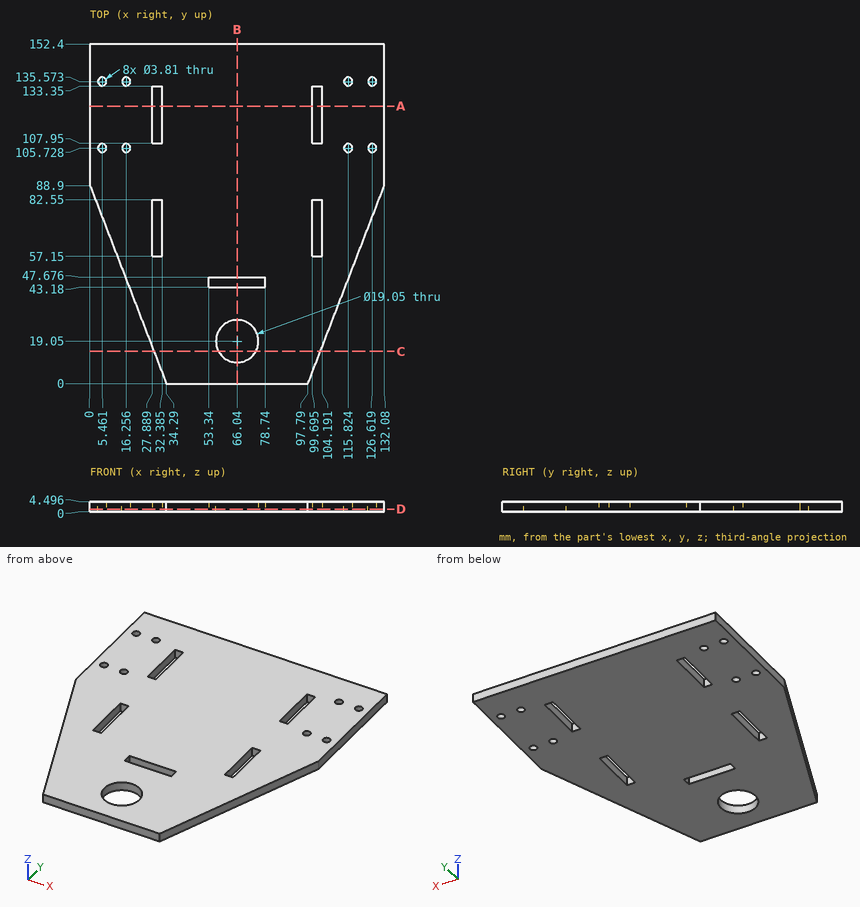
Geometry: see drawing. Coordinates: mm, zero at the bounding-box minimum. Round coordinates to 2 decimals unless told otherwise and drop trailing zeros. Write each loop counter-clockwise with the first axis right and the second up, starting at its lowest first coordinate (ties: lowest second). Pieces come first, ordered by that corner, then holes.
1) Cut plane B-B (x = 66.04). Return the cut outline in (y, z) (1 decimal).
2) Cut plane D-D (z = 1.15). Count the separate pieces of the cut face and the enclosed holes in it, then the cut area to 3 significant figures.
3) Cut plane A-A (y = 124.5). Return the cut outline in (x, z) (1 decimal).
4) Contact query for flat-ended pins moving along their axis: P1, Ø3.5, axis at x = 115.82, y = 105.73, coming from the +Z side; P2, Ø2, axis at y = 72.5, z = 2, coming from the -X side; P3, Ø2, axis at y = 75, z = 2.5, coming from the +X side (1 decimal); P4, Ø1.3, axis at y = 46.5, z = 3, coming from the -X side. Output: stop coordinate, or through.
5) Ray query, L1, parallel to X at y = 116, z = 0.5 (1 decimal); L2, parallel to X at y = 81, z = 2 (1 decimal); L3, parallel to Y at x = 60, z = 2 (1 decimal). Return the intervals inside material, ascending.
6) Cut plane C-C (y = 14.5). Return the cut outline in (x, z) (1 decimal).
Geometry says:
1. outline: (0, 0) - (9.5, 0) - (9.5, 4.5) - (0, 4.5) - close; (28.6, 0) - (43.2, 0) - (43.2, 4.5) - (28.6, 4.5) - close; (47.7, 0) - (152.4, 0) - (152.4, 4.5) - (47.7, 4.5) - close
2. separate pieces: 1
2. enclosed holes: 14
2. area: 16,100 mm2
3. outline: (0, 0) - (27.9, 0) - (27.9, 4.5) - (0, 4.5) - close; (32.4, 0) - (99.7, 0) - (99.7, 4.5) - (32.4, 4.5) - close; (104.2, 0) - (132.1, 0) - (132.1, 4.5) - (104.2, 4.5) - close
4. P1: passes through
4. P2: stops at x = 5.94
4. P3: stops at x = 127.1
4. P4: stops at x = 16.1
5. L1: x = 0 to 27.9, 32.4 to 99.7, 104.2 to 132.1
5. L2: x = 3 to 27.9, 32.4 to 99.7, 104.2 to 129
5. L3: y = 0 to 11.7, 26.4 to 43.2, 47.7 to 152.4
6. outline: (28.7, 0) - (57.7, 0) - (57.7, 4.5) - (28.7, 4.5) - close; (74.4, 0) - (103.4, 0) - (103.4, 4.5) - (74.4, 4.5) - close
